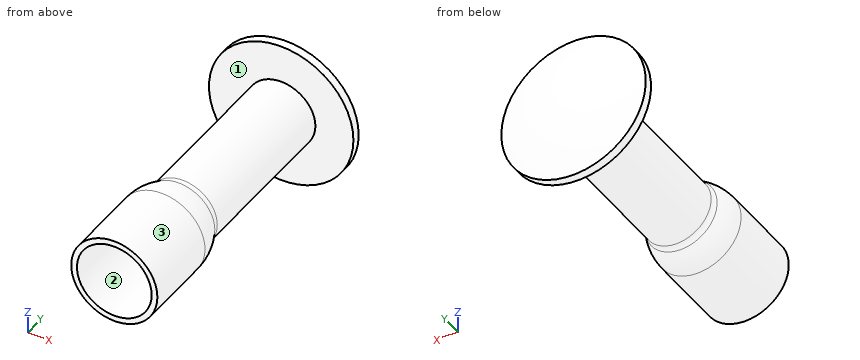
```python
from build123d import *


with BuildPart() as part:
    # Sketch1 → Revolve1 (revolve)
    with BuildSketch(Plane.XY):
        with BuildLine():
            Line((1.3, -6.804641901), (1.3, -9.525))
            Line((1.3, -9.525), (1.5, -9.525))
            Line((1.5, -9.525), (1.5, -6.804641901))
            ThreePointArc((1.5, -6.804641901), (1.437137063, -6.307148182), (1.2525, -5.84092838))
            ThreePointArc((1.2525, -5.84092838), (1.206340734, -5.72437343), (1.190625, -5.6))
            Line((1.190625, -5.6), (1.190625, 0))
            Line((1.190625, 0), (2.5146, 0))
            Line((2.5146, 0), (2.5146, 0.3))
            ThreePointArc((2.5146, 0.3), (1.283177404, 0.68329415), (0, 0.8128))
            Line((0, 0.8128), (0, 0))
            Line((0, 0), (0.990625, 0))
            Line((0.990625, 0), (0.990625, -5.6))
            ThreePointArc((0.990625, -5.6), (1.012627028, -5.774122801), (1.07725, -5.937299732))
            ThreePointArc((1.07725, -5.937299732), (1.243423357, -6.356897554), (1.3, -6.804641901))
        make_face()
    revolve(axis=Axis((0, 0.8128, 0), (0, -1, 0)))


solid = part.part
```
Could you check a few things on this model? Use its own coordinates, in mm. Face numbers are marked on the shaded views. Give positions to 0.01 mm unless a question says otherwise; leave off trailing zeros. Loops run counter-clockwise (first coordinate to the right, second up) from the corner with the lowest first, then second, coordinate; pieces in that order, holes last. Notation, with made-up numbers: (23, 35) -> (27, 35) arc R8 cw to (27, 46) -> close; hole circle Ø11 at (54, 5.25). An arc over 180 degrees is marked (long way). Put each result on its own line as item: value.
(1) Imagine slicing it at B-B on x = -1.75. Write out the boundary of the cut face in (y, z).
Computed:
outline: (0, -1.81) -> (0.3, -1.81) arc R6.18 ccw to (0.3, 1.81) -> (0, 1.81) -> close
(2) I'm going to push flat-ended pins straight in: pin 1 Ø3 at (x, y) = (-1, -2) entering from +Z; pin 2 Ø3 at (y, z) = (-6.5, 0) entering from -X; pin 3 Ø1.5 at (x, z) = (0.5, -1) entering from +Y. Where does each tip first touch, or does it pass through?
Computed:
pin 1: z = 1.19
pin 2: x = -1.5
pin 3: y = 0.8
(3) Please list where these lines run through material, in increasing order: probe 1 along Z at (x, y) = (0, -4.2); probe 2 along Z at (x, y) = (0, -7.6); probe 3 along X at (y, z) = (-8.75, 0.5). Write a range as [from, to].
Computed:
probe 1: [-1.19, -0.99], [0.99, 1.19]
probe 2: [-1.5, -1.3], [1.3, 1.5]
probe 3: [-1.41, -1.2], [1.2, 1.41]
(4) Imagine slicing it at A-A on y = -8. Write out the boundary of the cut face in (x, z).
Computed:
outline: circle Ø3 at (0, 0); hole circle Ø2.6 at (0, 0)
(5) Imagine slicing it at C-C on y = -1. Write out the boundary of the cut face in (x, z), plus the area to 3 significant figures.
Computed:
outline: circle Ø2.38 at (0, 0); hole circle Ø1.98 at (0, 0)
area: 1.37 mm^2
(6) Thinking about a two-plate mould opening in Z: for the marked faces 1, 2 and 3, which applies, pulls with the +Z half, pulls with the -Z half, needs draft (parallel to the pull), parting line crosses it, or undercut?
Computed:
face 1: needs draft
face 2: undercut
face 3: parting line crosses it
